Geometry check sheet. Reference: the model listing, model coordinates, mm. A direction names the side the tool comes from. Coordinates: 2 decimals unless noted, no trailing zeros. Write each loop counter-clockwise with the first axis right and the second up, starting at its lowest first coordinate (ties: lowest second). Pieces come first, ordered by that corner, then holes. Notation, with made-up numbers: M 3,37 L 30,37 A24 ccw 30,53 Z; hole C 30.5,47 d8. An arc over 180 degrees is marked long. Write item = value, one per line. Start each with the question number.
```python
from build123d import *

# Parameters (mm, degrees)
SKETCH1_R           = 53.18125
BOSS_EXTRUDE1_DEPTH = 50.8
SKETCH2_R           = 50.8
SKETCH2_R_2         = 50.4825
BOSS_EXTRUDE2_DEPTH = 2.54
SKETCH3_R           = 50.4825
CUT_EXTRUDE1_DEPTH  = 50.165
CUT_EXTRUDE1_DRAFT  = -5
SKETCH4_R           = 38.1
CUT_EXTRUDE3_DEPTH  = 3.175
SKETCH5_R           = 1.41224
CUT_EXTRUDE4_DEPTH  = 91.404745053
CIRPATTERN4_COUNT   = 8


with BuildPart() as part:
    # Sketch1 → Boss-Extrude1 (new body)
    with BuildSketch(Plane(origin=(0, 0, 0), x_dir=(1, 0, 0), z_dir=(0, 1, 0))):
        with Locations(Location((0, 0, 0), (0, 0, 270))):
            Circle(SKETCH1_R)
    extrude(amount=BOSS_EXTRUDE1_DEPTH)

    # Sketch2 → Boss-Extrude2 (add)
    with BuildSketch(Plane.XZ):
        with Locations(Location((0, 0, 0), (0, 0, 270))):
            Circle(SKETCH2_R)
        Circle(SKETCH2_R_2, mode=Mode.SUBTRACT)
        Circle(SKETCH2_R_2)
    extrude(amount=BOSS_EXTRUDE2_DEPTH)


with BuildPart() as cut_extrude1_tool:
    # Sketch3 → Cut-Extrude1 (with draft: the straight prism first)
    with BuildSketch(Plane(origin=(0, 50.8, 0), x_dir=(1, 0, 0), z_dir=(0, 1, 0))):
        Circle(SKETCH3_R)
    extrude(amount=-CUT_EXTRUDE1_DEPTH)
    # Cut-Extrude1: the draft: its side faces are tilted about the plane it starts from
    cut_extrude1_sides = [cut_extrude1_tool.faces().sort_by_distance(p)[0] for p in [
        (-50.4825, 25.7175, 0),
    ]]
    draft(cut_extrude1_sides, Plane(origin=(0, 50.8, 0), x_dir=(1, 0, 0), z_dir=(0, 1, 0)), CUT_EXTRUDE1_DRAFT)


with BuildPart() as part_1:
    add(part.part)

    # Cut-Extrude1: cut by cut_extrude1_tool
    add(cut_extrude1_tool.part, mode=Mode.SUBTRACT)

    # Sketch4 → Cut-Extrude3 (cut)
    with BuildSketch(Plane(origin=(0, 0.635, 0), x_dir=(1, 0, 0), z_dir=(0, 1, 0))):
        with Locations(Location((0, 0, 0), (0, 0, 270))):
            Circle(SKETCH4_R)
    extrude(amount=-CUT_EXTRUDE3_DEPTH, mode=Mode.SUBTRACT)

    # Sketch5 → Cut-Extrude4 (cut, through all)
    with BuildSketch(Plane(origin=(0, 0.635, 0), x_dir=(1, 0, 0), z_dir=(0, 1, 0))):
        with Locations(Location((-42.096815597, 0, 0), (0, 0, 270))):
            Circle(SKETCH5_R)
    cut_extrude4 = extrude(amount=-CUT_EXTRUDE4_DEPTH, mode=Mode.SUBTRACT)

    # CirPattern4: Cut-Extrude4 ×8 about axis
    cirpattern4_axis = Axis((0, 0, 0), (0, 1, 0))
    for i in range(1, CIRPATTERN4_COUNT):
        add(cut_extrude4.rotate(cirpattern4_axis, i * 360 / CIRPATTERN4_COUNT), mode=Mode.SUBTRACT)


solid = part_1.part
```
Q1. Gauge pin test, flat ends, axial feed: pin 1 (3 mm diameter, centred on y = 11, z = -10.5, fed in from -X); pin 2 (8 mm diameter, centred on x = -27, z = 25, fed in from -Y); pin 3 (3 mm diameter, centred on x = 0, z = 42.1, fed in from +Y) (3 decimals); pin 4 (2 mm diameter, centred on y = 3, z = 7, fed in from -X). Record the tip position at first contact, or that the pin passes through.
Q2. Draft check along X on faces 1 (the face through (-10.369, 20.495, 46.694)), 2 (the face through (-0.2, -0.9, 40.7)), 3 (the face through (-51.917, 25.044, -11.529)), 4 (the face through (-19, 50.8, 47)). Enter one of: pulls with the +X half, pulls with the -X half, needs draft (parallel to the pull), parting line crosses it, or undercut.
Q3. Cross-section at B-B on z = 0. Enter the section's corners in (x, y) (1 decimal).
Q4. Set-up check for faces 5 (the face through (-23.183, -0.93, -30.235)), 6 (the face through (-30.911, -1.252, 40.313)), 7 (the face through (-7, 0.635, -38)): record each of +Z, -Z, +X, -X, +Y, -Y from which the full face is reachable in a straight line by a thin tool's end or side.
Q5. Scan lines: L1, parallel to X at y = -0.8, z = 0; L2, parallel to Y at x = -35, z = -25 (3 decimals); L3, parallel to Z at x = 7.5, y = 35. Record each from-to range of solid material in increasing order.
Q6. Cross-section at A-A on x = 0. Enter the section's corners in (y, z) (1 decimal).
Q7. Cross-section at C-C on y = 15. Enter the section's corners in (x, z).
Values found:
q1.pin_1 = -52.41
q1.pin_2 = -2.54
q1.pin_3 = 0.635
q1.pin_4 = -52.84
q2.face_1 = undercut
q2.face_2 = undercut
q2.face_3 = parting line crosses it
q2.face_4 = needs draft
q3.outline = M -53.2,0 L -50.8,0 L -50.8,-2.5 L -43.5,-2.5 L -43.5,0.6 L -46.1,0.6 L -50.5,50.8 L -53.2,50.8 Z; M -40.7,-2.5 L -38.1,-2.5 L -38.1,0.6 L -40.7,0.6 Z; M 38.1,-2.5 L 40.7,-2.5 L 40.7,0.6 L 38.1,0.6 Z; M 43.5,-2.5 L 50.8,-2.5 L 50.8,0 L 53.2,0 L 53.2,50.8 L 50.5,50.8 L 46.1,0.6 L 43.5,0.6 Z
q4.face_5 = +Y, -Y
q4.face_6 = -Y
q4.face_7 = +Y
q5.L1 = -50.8 to -43.51, -40.68 to -38.1, 38.1 to 40.68, 43.51 to 50.8
q5.L2 = -2.54 to 0.635
q5.L3 = -52.65 to -48.52, 48.52 to 52.65
q6.outline = M -2.5,-50.8 L 0,-50.8 L 0,-53.2 L 50.8,-53.2 L 50.8,-50.5 L 0.6,-46.1 L 0.6,-43.5 L -2.5,-43.5 Z; M -2.5,-40.7 L 0.6,-40.7 L 0.6,-38.1 L -2.5,-38.1 Z; M -2.5,38.1 L 0.6,38.1 L 0.6,40.7 L -2.5,40.7 Z; M -2.5,43.5 L 0.6,43.5 L 0.6,46.1 L 50.8,50.5 L 50.8,53.2 L 0,53.2 L 0,50.8 L -2.5,50.8 Z
q7.outline = C 0,0 d106.36; hole C 0,0 d94.7
